```python
from build123d import *

# Parameters (mm, degrees)
SKETCH1_R           = 12.7
SKETCH1_R_2         = 6.35
BOSS_EXTRUDE1_DEPTH = 34.925
CHAMFER1_SIZE       = 2.5
SCALE1_SCALE        = 0.51948


with BuildPart() as part:
    # Sketch1 → Boss-Extrude1 (new, symmetric)
    with BuildSketch(Plane(origin=(0, 0, 0), x_dir=(1, 0, 0), z_dir=(0, 1, 0))):
        with Locations(Location((0, 0, 0), (0, 0, 270))):
            Circle(SKETCH1_R)
        with Locations(Location((0, 0, 0), (0, 0, 270))):
            Circle(SKETCH1_R_2, mode=Mode.SUBTRACT)
    extrude(amount=BOSS_EXTRUDE1_DEPTH, both=True)

    # Chamfer1
    chamfer1_edges = [part.edges().sort_by_distance(p)[0] for p in [
        (0, -34.925, -12.7),
        (0, 34.925, -12.7),
    ]]
    chamfer(chamfer1_edges, length=CHAMFER1_SIZE)


with BuildPart() as part_1:
    # Scale1: scaled about (0, 0, 0)
    add(part.part.scale(SCALE1_SCALE))


solid = part_1.part
```
Verification items for the finished model (mm, model axes). Give positions to 0.01 mm unless a question says otherwise; leave off trailing zeros. Order: outer loops, then holes, each group sorted by start corner. A loop starts at its lowest first (then second) coordinate and runs counter-clockwise, first axis right, second up. Notation, with made-up numbers: (-28.5, 6) -> (20.5, 6) arc R20 ccw to (20.5, 26) -> close; hole circle Ø11 at (62.5, 65). An arc over 180 degrees is marked (long way). One line per item, written item: value.
(1) Draft check along X on faces 1 (the face through (6.54, 0.24, -0.86)), 2 (the face through (3.27, -0.25, -0.43)), 3 (the face through (-3.5, 18.143, -0.1)). Enter one of: pulls with the +X half, pulls with the -X half, needs draft (parallel to the pull), parting line crosses it, or undercut.
Final values:
face 1: parting line crosses it
face 2: undercut
face 3: needs draft
(2) Sectioned sample at B-B on x = 0. Record the cut outline in (y, z), then the cut area to 3 significant figures.
Final values:
outline: (-18.14, -5.3) -> (-16.84, -6.6) -> (16.84, -6.6) -> (18.14, -5.3) -> (18.14, -3.3) -> (-18.14, -3.3) -> close; (-18.14, 3.3) -> (18.14, 3.3) -> (18.14, 5.3) -> (16.84, 6.6) -> (-16.84, 6.6) -> (-18.14, 5.3) -> close
area: 236 mm^2
(3) Scan lines: line 1 along X through (y, z) = (9.5, 0); line 2 along X through (y, z) = (-12, -2.5); line 3 along Z through (x, y) = (-1.75, 6.5). Record each from-to range of solid material in increasing order. Write a range as [from, to].
Final values:
line 1: [-6.6, -3.3], [3.3, 6.6]
line 2: [-6.11, -2.15], [2.15, 6.11]
line 3: [-6.36, -2.8], [2.8, 6.36]
(4) Sectioned sample at A-A on z = 0. Record the cut outline in (x, y), then the cut area to 3 significant figures.
Final values:
outline: (-6.6, -16.84) -> (-5.3, -18.14) -> (-3.3, -18.14) -> (-3.3, 18.14) -> (-5.3, 18.14) -> (-6.6, 16.84) -> close; (3.3, -18.14) -> (5.3, -18.14) -> (6.6, -16.84) -> (6.6, 16.84) -> (5.3, 18.14) -> (3.3, 18.14) -> close
area: 236 mm^2
(5) Sectioned sample at C-C on y = 15. Record the cut outline in (x, z).
Final values:
outline: circle Ø13.19 at (0, 0); hole circle Ø6.6 at (0, 0)
(6) Gauge pin test, flat ends, axial feed: pin 1 (1 mm diameter, centred on x = -4.5, y = -7.5, fed in from +Z); pin 2 (1.5 mm diameter, centred on x = -2.5, y = -8.5, fed in from +Z); pin 3 (1.5 mm diameter, centred on x = -1.5, y = -5.5, fed in from -Z). Record the tip position at first contact, or that the pin passes through.
Final values:
pin 1: z = 5.25
pin 2: z = 6.36
pin 3: z = -6.55
